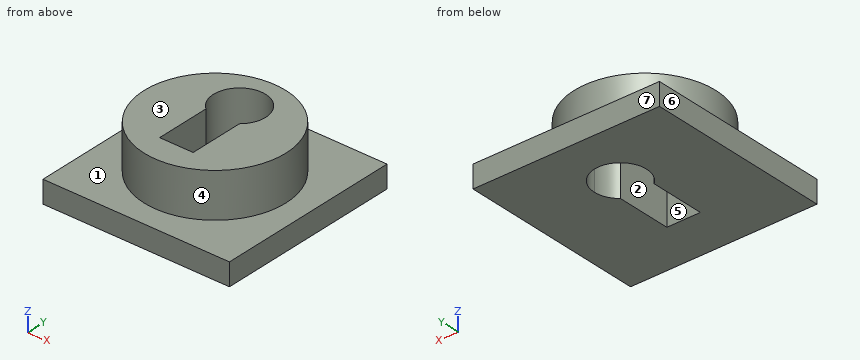
```python
from build123d import *

# Parameters (mm, degrees)
F0_W     = 25
F0_H     = 25
F1_DEPTH = 3
F2_R     = 9.5
F3_DEPTH = 6
F4_W     = 4.4934357473
F4_H     = 5.6233623327
F5_DEPTH = 9


with BuildPart() as f1:
    # F0 (on Top) → F1 (new body)
    with BuildSketch(Plane.XY):
        with Locations((-43.7815897167, 41.7574498571)):
            Rectangle(F0_W, F0_H)
    extrude(amount=F1_DEPTH)

    # F2 (on face) → F3 (join)
    with BuildSketch(Plane.XY.offset(3)):
        with Locations((-43.7815897167, 41.7574498571)):
            Circle(F2_R)
    extrude(amount=F3_DEPTH)

    # F4 (on face) → F5 (cut)
    with BuildSketch(Plane.XY.offset(9)):
        with Locations((-43.8689409503, 38.5465395694)):
            Rectangle(F4_W, F4_H)
        with BuildLine():
            ThreePointArc((-40.3680887796, 45.7565144868), (-45.3485456086, 48.9279885254), (-46.1156588239, 43.0735256877))
            Line((-46.1156588239, 43.0735256877), (-41.6222230767, 43.0735256877))
            Line((-41.6222230767, 43.0735256877), (-41.6222230767, 43.0720988624))
            ThreePointArc((-41.6222230767, 43.0720988624), (-40.6970849984, 44.2750506769), (-40.3680887796, 45.7565144868))
        make_face()
        with BuildLine():
            Line((-46.1156588239, 43.0735256877), (-46.1156588239, 41.3582207357))
            Line((-46.1156588239, 41.3582207357), (-41.6222230767, 41.3582207357))
            Line((-41.6222230767, 41.3582207357), (-41.6222230767, 43.0720988624))
            ThreePointArc((-41.6222230767, 43.0720988624), (-43.8692001537, 42.2565146632), (-46.1156588239, 43.0735256877))
        make_face()
        with BuildLine():
            Line((-41.6222230767, 43.0735256877), (-46.1156588239, 43.0735256877))
            ThreePointArc((-46.1156588239, 43.0735256877), (-43.8692001537, 42.2565146632), (-41.6222230767, 43.0720988624))
            Line((-41.6222230767, 43.0720988624), (-41.6222230767, 43.0735256877))
        make_face()
    extrude(amount=-F5_DEPTH, mode=Mode.SUBTRACT)


solid = f1.part
```
Geometry check sheet. Reference: the model listing, model coordinates, mm. Face numbers are marked on the shaded views. A direction names the side the tool comes from. Coordinates: 2 decimals unless noted, no trailing zeros. Write each loop counter-clockwise with the first axis right and the second up, starting at its lowest first coordinate (ties: lowest second). Pieces come first, ordered by that corner, then holes. Notation, with made-up numbers: M 35,-5 L 51,-5 A26 cw 51,34 Z; hole C 22,26.5 d5. An arc over 180 degrees is marked long. Answer as a JSON object with one key per item and string values.
1. Scan lines: L1, parallel to X at y = 41.75, z = 8; L2, parallel to Y at x = -43.75, z = 3.5; L3, parallel to Z at x = -36.5, y = 51.25. Record each from-to range of solid material in increasing order.
Answers below:
{"L1": "x = -53.28 to -46.12, -41.62 to -34.28", "L2": "y = 32.26 to 35.73, 49.25 to 51.26", "L3": "z = 0 to 3"}
2. Draft check along X on the marked faces 4, 5, 6 and 7. Enter one of: released by +X, released by -X, zero draft, split by the parting line, or undercut.
Answers below:
{"face 4": "split by the parting line", "face 5": "undercut", "face 6": "released by -X", "face 7": "zero draft"}
3. Section check C-C, the plane x = -46.5. Enter the section's corners in (y, z), plus the area to 3 significant figures.
Answers below:
{"outline": "M 29.26,0 L 43.45,0 L 43.45,9 L 32.65,9 L 32.65,3 L 29.26,3 Z; M 48.06,0 L 54.26,0 L 54.26,3 L 50.86,3 L 50.86,9 L 48.06,9 Z", "area": "143 mm²"}
4. Section check D-D, the plane x = -38. Enter the section's corners in (y, z).
Answers below:
{"outline": "M 29.26,0 L 54.26,0 L 54.26,3 L 49.3,3 L 49.3,9 L 34.22,9 L 34.22,3 L 29.26,3 Z"}
5. Tool access check on the marked faces 1, 2 and 3. Record the directions out of +Z, -Z, +X, -X, +Y, -Y that give a thin tool (end or side, any length) a straight path to the whole face; none if there is none.
Answers below:
{"face 1": "+Z", "face 2": "+Z, -Z", "face 3": "+Z, +X, -X, +Y, -Y"}
6. Section check B-B, the plane z = 0.75. Enter the section's corners in (x, y).
Answers below:
{"outline": "M -56.28,29.26 L -31.28,29.26 L -31.28,54.26 L -56.28,54.26 Z; hole M -46.12,35.73 L -41.62,35.73 L -41.62,43.07 A3.5 ccw long -46.12,43.07 Z"}
7. Section check A-A, the plane y = 38.25. Enter the section's corners in (x, z).
Answers below:
{"outline": "M -56.28,0 L -46.12,0 L -46.12,9 L -52.61,9 L -52.61,3 L -56.28,3 Z; M -41.62,0 L -31.28,0 L -31.28,3 L -34.95,3 L -34.95,9 L -41.62,9 Z"}
8. Go/stop test with flat-tipped pins: pin 1 Ø1.3 at (x, z) = (-44, 5.5) entering from +Y; pin 2 Ø1 at (x, z) = (-34.5, 5.5) entering from +Y. Record where each tip stops, or that it passes through.
Answers below:
{"pin 1": "stops at y = 51.26", "pin 2": "stops at y = 45.38"}
